from build123d import *

# Parameters (mm, degrees)
SKETCH1_W                  = 50.8
SKETCH1_H                  = 55.88
BOSS_EXTRUDE1_DEPTH        = 3.6
SKETCH2_W                  = 11.43
SKETCH2_H                  = 17.3228
BOSS_EXTRUDE2_DEPTH        = 0.5332
SKETCH3_W                  = 2.648
SKETCH3_H                  = 1.6
SKETCH4_W                  = 2.648
SKETCH4_H                  = 1.6
SKETCH5_W                  = 2.648
SKETCH5_H                  = 1.6
SKETCH6_W                  = 2.648
SKETCH6_H                  = 1.6
F_3_4_3_4_DIAMETER_HOLE1_D = 3.4


with BuildPart() as part:
    # Sketch1 → Boss-Extrude1 (new body)
    with BuildSketch(Plane.XY):
        with Locations((0, 2.54)):
            Rectangle(SKETCH1_W, SKETCH1_H)
    extrude(amount=-BOSS_EXTRUDE1_DEPTH)

    # Sketch2 → Boss-Extrude2 (add)
    with BuildSketch(Plane.XY):
        Rectangle(SKETCH2_W, SKETCH2_H)
    extrude(amount=BOSS_EXTRUDE2_DEPTH)

    # Sketch3 → Revolve1 (revolve)
    with BuildSketch(Plane.XZ.offset(-16.129)):
        with Locations((-11.376, 0.8)):
            Rectangle(SKETCH3_W, SKETCH3_H)
    revolve(axis=Axis((-12.7, 16.129, 1.6), (0, 0, -1)))

    # Sketch4 → Revolve2 (revolve)
    with BuildSketch(Plane.XZ.offset(16.129)):
        with Locations((-11.376, 0.8)):
            Rectangle(SKETCH4_W, SKETCH4_H)
    revolve(axis=Axis((-12.7, -16.129, 1.6), (0, 0, -1)))

    # Sketch5 → Revolve3 (revolve)
    with BuildSketch(Plane.XZ.offset(16.129)):
        with Locations((14.024, 0.8)):
            Rectangle(SKETCH5_W, SKETCH5_H)
    revolve(axis=Axis((12.7, -16.129, 1.6), (0, 0, -1)))

    # Sketch6 → Revolve4 (revolve)
    with BuildSketch(Plane.XZ.offset(-16.129)):
        with Locations((14.024, 0.8)):
            Rectangle(SKETCH6_W, SKETCH6_H)
    revolve(axis=Axis((12.7, 16.129, 1.6), (0, 0, -1)))

    # Ø3.4 (3.4) Diameter Hole1 (through all)
    with Locations(Plane.XY.offset(1.6)):
        with Locations((-12.7, -16.129), (12.7, -16.129), (12.7, 16.129), (-12.7, 16.129)):
            Hole(F_3_4_3_4_DIAMETER_HOLE1_D / 2)


solid = part.part
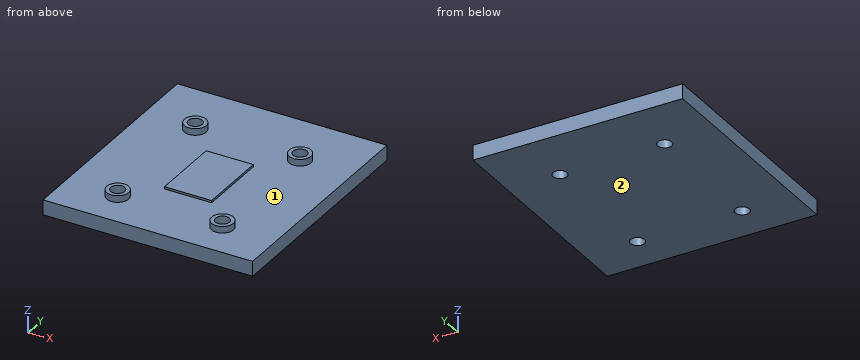
Work out the finished part from the listing and answer in its coordinate system (mm). Face numbers are marked on the shaded views. A direction names the side the tool comes from. Round coordinates to 2 decimals unless told otherwise and drop trailing zeros. Write each loop counter-clockwise with the first axis right and the second up, starting at its lowest first coordinate (ties: lowest second). Pieces come first, ordered by that corner, then holes.
1) A tool of negligible diameter and unlimited length cuts with its end or side. For the marked faces 1 and 2, from which of +Z, -Z, +X, -X, +Y, -Y can it reach the whole face along a straight path? Write none if from no direction.
2) A cutting plane is placed at D-D (x = -19.5). Give the vertices of the cut face in (y, z), plus the area to 3 significant figures.
3) Given pin 1 Ø8 at (x, y) = (8.5, -9.5) entering from +Z; pin 2 Ø8 at (x, y) = (9, 22) entering from +Z; pin 3 Ø5.5 at (x, y) = (12.7, -16.129) entering from +Z, each flat-ended and moving along its own axis, determine where each tip first touches the part or whether it passes through.
4) A cutting plane is placed at A-A (x = 12.7). Give the vertices of the cut face in (y, z), plus the area to 3 significant figures.
5) Straight lines are drawn through the part: line 1 (Y direction, x = 12.7, z = -1.2); line 2 (X direction, y = -16, z = -2.25); line 3 (X direction, y = -15, z = -3.25). For each, find the intervals that lie inside material, in ascending order.
6) A cutting plane is placed at C-C (x = 0.5). Give the vertices of the cut face in (y, z), plus the area to 3 significant figures.
7) A cutting plane is placed at B-B (y = -7). Give the vertices of the cut face in (x, z) (3 decimals), plus the area to 3 significant figures.
Completed:
1. face 1: +Z
1. face 2: -Z, +X, -X, +Y, -Y
2. outline: (-25.4, -3.6) - (30.48, -3.6) - (30.48, 0) - (-25.4, 0) - close
2. area: 201 mm2
3. pin 1: stops at z = 0.53
3. pin 2: stops at z = 0
3. pin 3: stops at z = 1.6
4. outline: (-25.4, -3.6) - (-17.83, -3.6) - (-17.83, 1.6) - (-18.78, 1.6) - (-18.78, 0) - (-25.4, 0) - close; (-14.43, -3.6) - (14.43, -3.6) - (14.43, 1.6) - (13.48, 1.6) - (13.48, 0) - (-13.48, 0) - (-13.48, 1.6) - (-14.43, 1.6) - close; (17.83, -3.6) - (30.48, -3.6) - (30.48, 0) - (18.78, 0) - (18.78, 1.6) - (17.83, 1.6) - close
4. area: 183 mm2
5. line 1: y = -25.4 to -17.83, -14.43 to 14.43, 17.83 to 30.48
5. line 2: x = -25.4 to -14.4, -11 to 11, 14.4 to 25.4
5. line 3: x = -25.4 to -13.97, -11.43 to 11.43, 13.97 to 25.4
6. outline: (-25.4, -3.6) - (30.48, -3.6) - (30.48, 0) - (8.66, 0) - (8.66, 0.53) - (-8.66, 0.53) - (-8.66, 0) - (-25.4, 0) - close
6. area: 210 mm2
7. outline: (-25.4, -3.6) - (25.4, -3.6) - (25.4, 0) - (5.715, 0) - (5.715, 0.533) - (-5.715, 0.533) - (-5.715, 0) - (-25.4, 0) - close
7. area: 189 mm2
